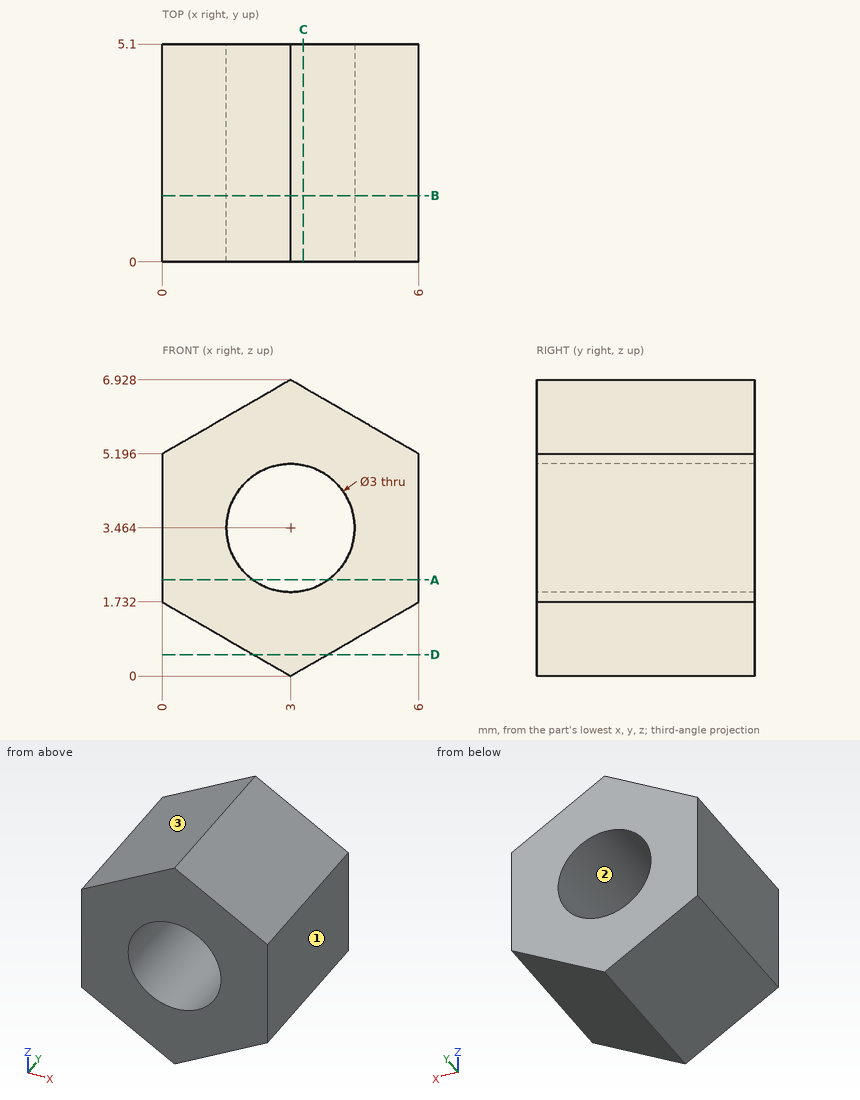
Geometry check sheet. Reference: drawing and pictorial views, mm from the part's lowest x, y, z. Round coordinates to 2 decimals unless told otherwise and drop trailing zeros. Loops run counter-clockwise (first coordinate to the right, second up) from the corner with the lowest first, then second, coordinate; pieces in that order, holes last. Notation, with made-up numbers: (-25, 2.25) -> (25, 2.25) arc R29 cw to (25, 41.25) -> close; hole circle Ø10 at (67.5, 6). An arc over 180 degrees is marked (long way). Answer as a JSON object with one key per item and string values.
Q1. Section check B-B (y = 1.55). Record the boundary of the cut face in (x, z), then the cut area to 3 significant figures.
Data:
{"outline": "(0, 1.73) -> (3, 0) -> (6, 1.73) -> (6, 5.2) -> (3, 6.93) -> (0, 5.2) -> close; hole circle Ø3 at (3, 3.46)", "area": "24.1 mm2"}
Q2. Go/stop test with a flat-tipped pin: P1, Ø1.5, axis at x = 1.5, y = 2.5, coming from the -Z side. Record where the tip stops, or that it passes through.
Data:
{"P1": "stops at z = 0.43"}
Q3. Section check C-C (x = 3.3). Record the boundary of the cut face in (y, z) (1 decimal).
Data:
{"outline": "(0, 0.2) -> (5.1, 0.2) -> (5.1, 2) -> (0, 2) -> close; (0, 4.9) -> (5.1, 4.9) -> (5.1, 6.8) -> (0, 6.8) -> close"}
Q4. Section check A-A (z = 2.25). Record the boundary of the cut face in (x, y), then the cut area to 3 significant figures.
Data:
{"outline": "(0, 0) -> (2.12, 0) -> (2.12, 5.1) -> (0, 5.1) -> close; (3.88, 0) -> (6, 0) -> (6, 5.1) -> (3.88, 5.1) -> close", "area": "21.6 mm2"}
Q5. Draft check along X on the marked faces 1, 2 and 3. Enter one of: pulls with the +X half, pulls with the -X half, needs draft (parallel to the pull), parting line crosses it, or undercut.
Data:
{"face 1": "pulls with the +X half", "face 2": "undercut", "face 3": "pulls with the -X half"}
Q6. Scan lines: line 1 (X direction, y = 3.05, z = 3.25) (1 decimal); line 2 (Z direction, x = 3.85, y = 3.3); line 3 (X direction, y = 2.4, z = 4.25). Record each from-to range of solid material in increasing order. Write a range as from..to.
Data:
{"line 1": "x = 0..1.5, 4.5..6", "line 2": "z = 0.49..2.23, 4.7..6.44", "line 3": "x = 0..1.72, 4.28..6"}
Q7. Section check D-D (z = 0.5). Record the boundary of the cut face in (x, y).
Data:
{"outline": "(2.13, 0) -> (3.87, 0) -> (3.87, 5.1) -> (2.13, 5.1) -> close"}
